```python
from build123d import *

# Parameters (mm, degrees)
F0_W     = 213
F0_H     = 46.5
F0_W_2   = 22.5
F0_H_2   = 40.5
F1_DEPTH = 2
F2_R     = 1


# Not quite as in the source:
# - a feature names something its author has since deleted; it is built from what else it names


with BuildPart() as f1:
    # F0 (on Front) → F1 (new body)
    with BuildSketch(Plane.XZ):
        with Locations((1.4150981574, 5.1332409506)):
            Rectangle(F0_W, F0_H)
        with Locations((-91.3349018426, 5.1332409506)):
            Rectangle(F0_W_2, F0_H_2, mode=Mode.SUBTRACT)
        with Locations((-64.8349018426, 5.1332409506)):
            Rectangle(F0_W_2, F0_H_2, mode=Mode.SUBTRACT)
        with Locations((-38.3349018426, 5.1332409506)):
            Rectangle(F0_W_2, F0_H_2, mode=Mode.SUBTRACT)
        with Locations((-11.8349018426, 5.1332409506)):
            Rectangle(F0_W_2, F0_H_2, mode=Mode.SUBTRACT)
        with Locations((14.6650981574, 5.1332409506)):
            Rectangle(F0_W_2, F0_H_2, mode=Mode.SUBTRACT)
        with Locations((41.1650981574, 5.1332409506)):
            Rectangle(F0_W_2, F0_H_2, mode=Mode.SUBTRACT)
        with Locations((67.6650981574, 5.1332409506)):
            Rectangle(F0_W_2, F0_H_2, mode=Mode.SUBTRACT)
        with Locations((94.1650981574, 5.1332409506)):
            Rectangle(F0_W_2, F0_H_2, mode=Mode.SUBTRACT)
    extrude(amount=F1_DEPTH)

    # F2
    f2_edges = [f1.edges().sort_by_distance(p)[0] for p in [
        (-80.084902, -1, 25.383241),
        (-102.584902, -1, 25.383241),
        (-80.084902, -1, -15.116759),
        (-102.584902, -1, -15.116759),
        (107.915098, -1, 28.383241),
        (107.915098, -1, -18.116759),
        (-105.084902, -1, 28.383241),
        (-105.084902, -1, -18.116759),
        (-76.084902, -1, 25.383241),
        (-49.584902, -1, 25.383241),
        (-23.084902, -1, 25.383241),
        (3.415098, -1, 25.383241),
        (29.915098, -1, 25.383241),
        (56.415098, -1, 25.383241),
        (82.915098, -1, 25.383241),
        (-53.584902, -1, 25.383241),
        (-27.084902, -1, 25.383241),
        (-0.584902, -1, 25.383241),
        (25.915098, -1, 25.383241),
        (52.415098, -1, 25.383241),
        (78.915098, -1, 25.383241),
        (105.415098, -1, 25.383241),
        (-76.084902, -1, -15.116759),
        (-49.584902, -1, -15.116759),
        (-23.084902, -1, -15.116759),
        (3.415098, -1, -15.116759),
        (29.915098, -1, -15.116759),
        (56.415098, -1, -15.116759),
        (82.915098, -1, -15.116759),
        (-53.584902, -1, -15.116759),
        (-27.084902, -1, -15.116759),
        (-0.584902, -1, -15.116759),
        (25.915098, -1, -15.116759),
        (52.415098, -1, -15.116759),
        (78.915098, -1, -15.116759),
        (105.415098, -1, -15.116759),
    ]]
    fillet(f2_edges, radius=F2_R)


solid = f1.part
```
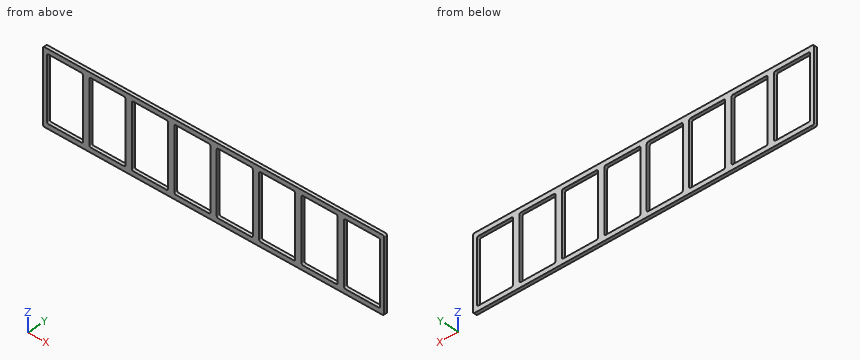
Model file for the job. Use its own axes, mm. Coordinates: 2 decimals unless noted, no trailing zeros. Order: outer loops, then holes, each group sorted by start corner. A loop starts at its lowest first (then second) coordinate and runs counter-clockwise, first axis right, second up. Notation, with made-up numbers: (36, 11.25) -> (50, 11.25) arc R35 ccw to (50, 49.25) -> close; hole circle Ø2 at (64, -32.5). An arc over 180 degrees is marked (long way). Answer as a JSON object with one key per item and string values. Group by question number.
1) Cut at B-B, the plane z = 9.5. Count the separate pieces of the cut face and the enclosed holes in it, then the cut area to 3 significant figures.
2) Cut at A-A, the plane x = 59.5. Write the cut outline in (y, z).
3) Drill centre line: L1, parallel to Z at x = -44.5, y = -0.05. Where is it in solid material? Low to high.
Check values:
{
 "1": {"separate pieces": "9", "enclosed holes": "0", "area": "66.0 mm²"},
 "2": {"outline": "(-2, -18.12) -> (0, -18.12) -> (0, -15.12) -> (-2, -15.12) -> close; (-2, 25.38) -> (0, 25.38) -> (0, 28.38) -> (-2, 28.38) -> close"},
 "3": {"L1": "z = -18.12 to -15.12, 25.38 to 28.38"}
}
